Geometry check sheet. Reference: the model listing, model coordinates, mm. Round coordinates to 2 decimals unless told otherwise and drop trailing zeros. Order: outer loops, then holes, each group sorted by start corner. A loop starts at its lowest first (then second) coordinate and runs counter-clockwise, first axis right, second up. Notation, with made-up numbers: (44, 63.5) -> (85, 63.5) arc R20 cw to (85, 75.5) -> close; hole circle Ø11 at (64, 40.25). An arc over 180 degrees is marked (long way). Use a Markdown table: item, result. Add a question column.
Item 1: Sectioned sample at C-C, the plane x = 35. Record the cut outline in (y, z), and give its area (3 significant figures).
Item 2: Sectioned sample at D-D, the plane y = 18.5. Record the cut outline in (x, z), and give its area (3 significant figures).
Item 3: Gauge pin test, flat end, axial feed: pin 1 Ø2 at (y, z) = (9.5, 1) entering from -X. Record the tip position at first contact, or that the pin passes through.
Item 4: Sectioned sample at A-A, the plane x = 80.5. Record the cut outline in (y, z).
Item 5: Sectioned sample at B-B, the plane z = 0.75. State how many separate pieces and enclosed holes the cut face has, and give its area (3 significant figures).
Item 6: Material ranges on probe 1 along Y at (x, z) = (35, 2); probe 2 along Y at (x, z) = (97, 1.6); probe 3 along Y at (x, z) = (145, 2.9), recorded low to high. Write a range as [from, to].
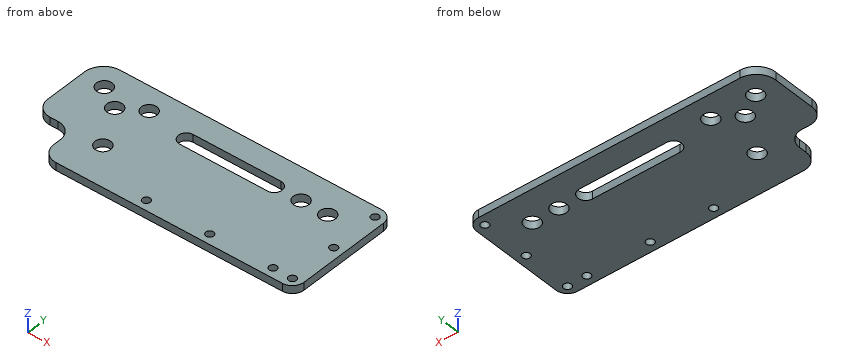
from build123d import *

# Parameters (mm, degrees)
SKETCH1_R           = 4
SKETCH1_R_2         = 2
BOSS_EXTRUDE1_DEPTH = 4


with BuildPart() as part:
    # Sketch1 → Boss-Extrude1 (new body)
    with BuildSketch(Plane.XY):
        with BuildLine():
            Line((28, 0), (140, 0))
            Line((140, 0), (144, 0))
            ThreePointArc((144, 0), (148.242640687, 1.757359313), (150, 6))
            Line((150, 6), (150, 54))
            ThreePointArc((150, 54), (148.242640687, 58.242640687), (144, 60))
            Line((144, 60), (140, 60))
            Line((140, 60), (10, 60))
            ThreePointArc((10, 60), (2.928932188, 57.071067812), (0, 50))
            Line((0, 50), (0, 28))
            ThreePointArc((0, 28), (2.343145751, 22.343145751), (8, 20))
            Line((8, 20), (12, 20))
            ThreePointArc((12, 20), (17.656854249, 17.656854249), (20, 12))
            Line((20, 12), (20, 8))
            ThreePointArc((20, 8), (22.343145751, 2.343145751), (28, 0))
        make_face()
        with Locations((35, 20)):
            Circle(SKETCH1_R, mode=Mode.SUBTRACT)
        with Locations((116.264838239, 44)):
            Circle(SKETCH1_R, mode=Mode.SUBTRACT)
        with Locations((129.947688147, 44)):
            Circle(SKETCH1_R, mode=Mode.SUBTRACT)
        with Locations((12, 48)):
            Circle(SKETCH1_R, mode=Mode.SUBTRACT)
        with Locations((23.5, 40.719874776)):
            Circle(SKETCH1_R, mode=Mode.SUBTRACT)
        with Locations((35, 48)):
            Circle(SKETCH1_R, mode=Mode.SUBTRACT)
        with Locations((135, 5)):
            Circle(SKETCH1_R_2, mode=Mode.SUBTRACT)
        with Locations((102.5, 5)):
            Circle(SKETCH1_R_2, mode=Mode.SUBTRACT)
        with Locations((70, 5)):
            Circle(SKETCH1_R_2, mode=Mode.SUBTRACT)
        with Locations((145, 54.898560305)):
            Circle(SKETCH1_R_2, mode=Mode.SUBTRACT)
        with Locations((145, 29.898560305)):
            Circle(SKETCH1_R_2, mode=Mode.SUBTRACT)
        with Locations((145, 4.898560305)):
            Circle(SKETCH1_R_2, mode=Mode.SUBTRACT)
        with BuildLine():
            Line((57.5, 48), (102.5, 48))
            ThreePointArc((102.5, 48), (106.5, 44), (102.5, 40))
            Line((102.5, 40), (57.5, 40))
            ThreePointArc((57.5, 40), (53.5, 44), (57.5, 48))
        make_face(mode=Mode.SUBTRACT)
    extrude(amount=BOSS_EXTRUDE1_DEPTH)


solid = part.part
Found:
| question | item | result |
|---|---|---|
| 1 | outline | (0, 0) -> (16, 0) -> (16, 4) -> (0, 4) -> close; (24, 0) -> (44, 0) -> (44, 4) -> (24, 4) -> close; (52, 0) -> (60, 0) -> (60, 4) -> (52, 4) -> close |
| 1 | area | 176 mm2 |
| 2 | outline | (16.66, 0) -> (31.29, 0) -> (31.29, 4) -> (16.66, 4) -> close; (38.71, 0) -> (150, 0) -> (150, 4) -> (38.71, 4) -> close |
| 2 | area | 504 mm2 |
| 3 | pin 1 | stops at x = 20 |
| 4 | outline | (0, 0) -> (40, 0) -> (40, 4) -> (0, 4) -> close; (48, 0) -> (60, 0) -> (60, 4) -> (48, 4) -> close |
| 5 | separate pieces | 1 |
| 5 | enclosed holes | 13 |
| 5 | area | 7,760 mm2 |
| 6 | probe 1 | y = [0, 16], [24, 44], [52, 60] |
| 6 | probe 2 | y = [0, 40], [48, 60] |
| 6 | probe 3 | y = [0.08, 2.9], [6.9, 27.9], [31.9, 52.9], [56.9, 59.92] |
